Part model, mm, in its own coordinate system. A direction names the side the tool comes from. Round coordinates to 2 decimals unless told otherwise and drop trailing zeros. Order: outer loops, then holes, each group sorted by start corner. A loop starts at its lowest first (then second) coordinate and runs counter-clockwise, first axis right, second up. Notation, with made-up numbers: (1.5, 64) -> (49.5, 64) arc R11 cw to (49.5, 68) -> close; hole circle Ø9 at (41, 47.5). An arc over 180 degrees is marked (long way). Return JSON: item names as keys, results as strings. Group by question number.
from build123d import *

# Parameters (mm, degrees)
SKETCH1_W           = 85
SKETCH1_H           = 25
BOSS_EXTRUDE1_DEPTH = 3
SKETCH2_W           = 83
SKETCH2_H           = 3.75
SKETCH2_H_2         = 2
SKETCH2_H_3         = 1.75
CUT_EXTRUDE1_DEPTH  = 2.5
SKETCH3_R           = 1.75
CUT_EXTRUDE2_DEPTH  = 45.401576549
SKETCH4_W           = 60
SKETCH4_H           = 5
CUT_EXTRUDE3_DEPTH  = 45.401576549
FILLET1_R           = 1
FILLET2_R           = 2


with BuildPart() as part:
    # Sketch1 → Boss-Extrude1 (new body)
    with BuildSketch(Plane(origin=(0, 0, 0), x_dir=(1, 0, 0), z_dir=(0, 1, 0))):
        Rectangle(SKETCH1_W, SKETCH1_H)
    extrude(amount=BOSS_EXTRUDE1_DEPTH)

    # Sketch2 → Cut-Extrude1 (cut)
    with BuildSketch(Plane(origin=(0, 3, 0), x_dir=(1, 0, 0), z_dir=(0, 1, 0))):
        with Locations((0, -9.625)):
            Rectangle(SKETCH2_W, SKETCH2_H)
        with Locations((0, -1.25)):
            Rectangle(SKETCH2_W, SKETCH2_H_2)
        with Locations((0, 2.875)):
            Rectangle(SKETCH2_W, SKETCH2_H_3)
    extrude(amount=-CUT_EXTRUDE1_DEPTH, mode=Mode.SUBTRACT)

    # Sketch3 → Cut-Extrude2 (cut, through all)
    with BuildSketch(Plane(origin=(0, 3, 0), x_dir=(1, 0, 0), z_dir=(0, 1, 0))):
        with Locations(Location((-38.5, 8.5, 0), (0, 0, 270))):
            Circle(SKETCH3_R)
        with Locations(Location((38.5, 8.5, 0), (0, 0, 90))):
            Circle(SKETCH3_R)
        with Locations(Location((-29, -5, 0), (0, 0, 270))):
            Circle(SKETCH3_R)
        with Locations(Location((29, -5, 0), (0, 0, 90))):
            Circle(SKETCH3_R)
    extrude(amount=-CUT_EXTRUDE2_DEPTH, mode=Mode.SUBTRACT)

    # Sketch4 → Cut-Extrude3 (cut, through all)
    with BuildSketch(Plane(origin=(0, 3, 0), x_dir=(1, 0, 0), z_dir=(0, 1, 0))):
        with Locations((0, 5.75)):
            Rectangle(SKETCH4_W, SKETCH4_H)
    extrude(amount=-CUT_EXTRUDE3_DEPTH, mode=Mode.SUBTRACT)

    # Fillet1
    fillet1_edges = [part.edges().sort_by_distance(p)[0] for p in [
        (30, 0.25, -3.25),
        (30, 1.5, -8.25),
        (-30, 1.5, -8.25),
        (-30, 0.25, -3.25),
    ]]
    fillet(fillet1_edges, radius=FILLET1_R)

    # Fillet2
    fillet2_edges = [part.edges().sort_by_distance(p)[0] for p in [
        (-42.5, 1.5, -12.5),
        (42.5, 1.5, -12.5),
        (42.5, 1.5, 12.5),
        (-42.5, 1.5, 12.5),
    ]]
    fillet(fillet2_edges, radius=FILLET2_R)


solid = part.part
(1) Saw through at B-B, the plane z = -5. List the corners of the cut face in (x, y).
(2) Probe L1, parallel to Z at x = 7.5, y = 0.8; L2, parallel to Z at x = -36, y = 2.05; L3, parallel to Z at x = 38.5, y = 0.7. List the from-to ranges inside material, lowest first. Write a range as [from, to].
(3) Saw through at C-C, the plane y = 1.45. State how many separate pieces and enclosed holes the cut face has, and give its area (3 significant figures).
(4) Mould opens along X. For faces 4 (the flat face through (-1, 1, 12.5)), 5 (the cylindrical face through (-41.93, 1.52, 11.9)), 6 (the flat face through (-36, 2, -3.75)) say: pulls with the +X half, pulls with the -X half, needs draft (parallel to the pull), parting line crosses it, or undercut.
(5) Saw through at D-D, the plane z = 5. List the corners of the cut face in (x, y), and give its area (3 significant figures).
(6) Tool access for faces 1 (the flat face through (-1, 0, 0)), 2 (the flat face through (0, 2, -8.25)), 3 (the flat face through (-1, 0.5, 1)): list every direction of +Z, -Z, +X, -X, +Y, -Y with a clear straight run to the whole face (end or side of a thin tool).
(7) Saw through at A-A, the plane x = 16. List the corners of the cut face in (y, z).
(8) Pin check, flat tips, straight feed: P1, Ø3, axis at x = -38.5, z = -8.5, coming from the -Y side; P2, Ø1.9, axis at x = -2, z = 9, coming from the +Y side. Stop position of each tip, or through.
Results are:
{
 "1": {"outline": "(-42.5, 0) -> (-30, 0) -> (-30, 3) -> (-42.5, 3) -> close; (30, 0) -> (42.5, 0) -> (42.5, 3) -> (30, 3) -> close"},
 "2": {"L1": "z = [-12.5, -8.25], [-2, 0.25], [2.25, 7.75], [11.5, 12.5]", "L2": "z = [-12.5, -3.75], [-2, 0.25], [2.25, 7.75], [11.5, 12.5]", "L3": "z = [-12.5, -10.25], [-6.75, -3.75], [-2, 0.25], [2.25, 7.75], [11.5, 12.5]"},
 "3": {"separate pieces": "1", "enclosed holes": "7", "area": "1,190 mm^2"},
 "4": {"face 4": "needs draft", "face 5": "pulls with the -X half", "face 6": "undercut"},
 "5": {"outline": "(-42.5, 0) -> (-30.75, 0) -> (-30.75, 3) -> (-42.5, 3) -> close; (-27.25, 0) -> (27.25, 0) -> (27.25, 3) -> (-27.25, 3) -> close; (30.75, 0) -> (42.5, 0) -> (42.5, 3) -> (30.75, 3) -> close", "area": "234 mm^2"},
 "6": {"face 1": "+Z, -Z, +X, -X, -Y", "face 2": "+Y, -Y", "face 3": "+Y"},
 "7": {"outline": "(0, -12.5) -> (3, -12.5) -> (3, -8.25) -> (0, -8.25) -> close; (0, -3.25) -> (0.5, -3.25) -> (0.5, -2) -> (3, -2) -> (3, 0.25) -> (0.5, 0.25) -> (0.5, 2.25) -> (3, 2.25) -> (3, 7.75) -> (0.5, 7.75) -> (0.5, 11.5) -> (3, 11.5) -> (3, 12.5) -> (0, 12.5) -> close"},
 "8": {"P1": "passes through", "P2": "stops at y = 0.5"}
}
